CAD build for the part. Positions are in the model's coordinates, mm. A direction names the side the tool comes from. Round coordinates to 2 decimals unless told otherwise and drop trailing zeros. Loops run counter-clockwise (first coordinate to the right, second up) from the corner with the lowest first, then second, coordinate; pieces in that order, holes last.
```python
from build123d import *

# Parameters (mm, degrees)
F0_W     = 90
F0_H     = 60
F1_DEPTH = 60
F2_W     = 60
F2_H     = 60
F3_DEPTH = 30
F4_R     = 10
F5_DEPTH = 55.20023


with BuildPart() as f1:
    # F0 (on Front) → F1 (new body)
    with BuildSketch(Plane.XZ):
        with Locations((3.869617, 6.589345)):
            Rectangle(F0_W, F0_H)
    extrude(amount=F1_DEPTH)

    # F2 (on face) → F3 (cut)
    with BuildSketch(Plane.XY.offset(36.589345)):
        with Locations((18.869617, -30)):
            Rectangle(F2_W, F2_H)
    extrude(amount=-F3_DEPTH, mode=Mode.SUBTRACT)

    # F4 (on face) → F5 (cut)
    with BuildSketch(Plane.XY.offset(6.589345)):
        with Locations((28.869617, -30)):
            Circle(F4_R)
    extrude(amount=-F5_DEPTH, mode=Mode.SUBTRACT)


solid = f1.part
```
Item 1: Cut at D-D, the plane y = -55.5. Give the cut face in (x, z), plus the area to 3 significant figures.
Answers follow:
outline: (-41.13, -23.41) - (48.87, -23.41) - (48.87, 6.59) - (-11.13, 6.59) - (-11.13, 36.59) - (-41.13, 36.59) - close
area: 3,600 mm2
Item 2: Flat gauge pin, fed straight in: P1, Ø10, axis at y = -46.5, z = 19, coming from the +X side. Where does the tip first touch, or does it go through?
Answers follow:
P1: stops at x = -11.13
Item 3: Probe line 1 (Y direction, x = 28.5, z = -13.5); line 2 (Z direction, x = 20, y = -17); line 3 (Y direction, x = 36, z = -9). List the from-to ranges inside material, lowest first.
Answers follow:
line 1: y = -60 to -39.99, -20.01 to 0
line 2: z = -23.41 to 6.59
line 3: y = -60 to -37.01, -22.99 to 0
Item 4: 3-axis set-ups, long thin cutter, end or side, ignore diameter. For faces 1 (the flat face through (-7, 0, 0)), 2 (the flat face through (18, -30, 6.589)): which of +Z, -Z, +X, -X, +Y, -Y reach the whole face in a straight line?
Answers follow:
face 1: +Z, -Z, +X, -X, +Y
face 2: +Z, +X, +Y, -Y
Item 5: Cut at C-C, the plane x = 35. Give the cut face in (y, z).
Answers follow:
outline: (-60, -23.41) - (-37.9, -23.41) - (-37.9, 6.59) - (-60, 6.59) - close; (-22.1, -23.41) - (0, -23.41) - (0, 6.59) - (-22.1, 6.59) - close
Item 6: Cut at A-A, the plane y = -30. Give the cut face in (x, z).
Answers follow:
outline: (-41.13, -23.41) - (18.87, -23.41) - (18.87, 6.59) - (-11.13, 6.59) - (-11.13, 36.59) - (-41.13, 36.59) - close; (38.87, -23.41) - (48.87, -23.41) - (48.87, 6.59) - (38.87, 6.59) - close
Item 7: Cut at B-B, the plane z = 0.5. Give the cut face in (x, y), plus the area to 3 significant figures.
Answers follow:
outline: (-41.13, -60) - (48.87, -60) - (48.87, 0) - (-41.13, 0) - close; hole circle Ø20 at (28.87, -30)
area: 5,090 mm2
Item 8: Two-plate mould, pull along X, no slides. Class faces 3 (the flat face through (-41.13, -30, 6)), 4 (the cylindrical face through (33.484, -38.872, -8.201)), 5 (the flat face through (-11.13, -30, 22)), 6 (the flat face through (-26, -30, 36.589)): released by +X, released by -X, zero draft, split by the parting line, or undercut.
Answers follow:
face 3: released by -X
face 4: undercut
face 5: released by +X
face 6: zero draft
